CAD build for the part. Positions are in the model's coordinates, mm. A direction names the side the tool comes from. Round coordinates to 2 decimals unless told otherwise and drop trailing zeros. Order: outer loops, then holes, each group sorted by start corner. A loop starts at its lowest first (then second) coordinate and runs counter-clockwise, first axis right, second up. Notation, with made-up numbers: M 11,20 L 15,20 A17 ccw 15,33 Z; hole C -19,72 d7. An arc over 180 degrees is marked long. Answer as a JSON object with one key per item and string values.
```python
from build123d import *

# Parameters (mm, degrees)
EXTRUDE_1_DEPTH     = 100
FILLET_1_R          = 2
SKETCH_2_R          = 2.2
CUT_EXTRUDE_1_DEPTH = 12
CHAMFER_1_SIZE      = 0.4


with BuildPart() as part:
    # Эскиз1 → Бобышка-Вытянуть1 (new body)
    with BuildSketch(Plane.XY):
        Polygon((0, 125), (-36.084391824, 62.5), (-108.253175473, 62.5), (-72.168783649, 0), (-108.253175473, -62.5), (-36.084391824, -62.5), (0, -125), (36.084391824, -62.5), (108.253175473, -62.5), (72.168783649, 0), (108.253175473, 62.5), (36.084391824, 62.5), align=None)
        Polygon((0, 105), (-24.537386441, 62.5), (24.537386441, 62.5), align=None, mode=Mode.SUBTRACT)
        Polygon((-90.932667397, -52.5), (-41.857894516, -52.5), (-66.395280957, -10), align=None, mode=Mode.SUBTRACT)
        Polygon((90.932667397, -52.5), (66.395280957, -10), (41.857894516, -52.5), align=None, mode=Mode.SUBTRACT)
        Polygon((-90.932667397, 52.5), (-41.857894516, 52.5), (-66.395280957, 10), align=None, mode=Mode.SUBTRACT)
        Polygon((90.932667397, 52.5), (66.395280957, 10), (41.857894516, 52.5), align=None, mode=Mode.SUBTRACT)
        Polygon((0, -105), (-24.537386441, -62.5), (24.537386441, -62.5), align=None, mode=Mode.SUBTRACT)
        Polygon((-30.310889132, 52.5), (30.310889132, 52.5), (60.621778265, 0), (30.310889132, -52.5), (-30.310889132, -52.5), (-60.621778265, 0), align=None, mode=Mode.SUBTRACT)
    extrude(amount=EXTRUDE_1_DEPTH)

    # Скругление1
    fillet_1_edges = [part.edges().sort_by_distance(p)[0] for p in [
        (108.253175473, 62.5, 50),
        (108.253175473, -62.5, 50),
        (0, -125, 50),
        (-108.253175473, -62.5, 50),
        (-108.253175473, 62.5, 50),
        (0, 125, 50),
    ]]
    fillet(fillet_1_edges, radius=FILLET_1_R)

    # Эскиз2 → Вырез-Вытянуть1 (cut)
    with BuildSketch(Plane.XY.offset(100)):
        with Locations((0, 115)):
            Circle(SKETCH_2_R)
        with Locations((-99.592921435, -57.5)):
            Circle(SKETCH_2_R)
        with Locations((99.592921435, -57.5)):
            Circle(SKETCH_2_R)
        with Locations((-33.197640478, 57.5)):
            Circle(SKETCH_2_R)
        with Locations((33.197640478, 57.5)):
            Circle(SKETCH_2_R)
        with Locations(Location((-99.592921435, 57.5, 0), (0, 0, 180))):
            Circle(SKETCH_2_R)
        with Locations(Location((99.592921435, 57.5, 0), (0, 0, 180))):
            Circle(SKETCH_2_R)
        with Locations(Location((33.197640478, -57.5, 0), (0, 0, 180))):
            Circle(SKETCH_2_R)
        with Locations(Location((-33.197640478, -57.5, 0), (0, 0, 180))):
            Circle(SKETCH_2_R)
        with Locations(Location((0, -115, 0), (0, 0, 180))):
            Circle(SKETCH_2_R)
        with Locations((-66.395280957, 0)):
            Circle(SKETCH_2_R)
        with Locations((66.395280957, 0)):
            Circle(SKETCH_2_R)
    extrude(amount=-CUT_EXTRUDE_1_DEPTH, mode=Mode.SUBTRACT)

    # Фаска1
    chamfer_1_edges = [part.edges().sort_by_distance(p)[0] for p in [
        (-2.2, 115, 100),
        (64.195280957, 0, 100),
        (-68.595280957, 0, 100),
        (2.2, -115, 100),
        (-101.792921435, -57.5, 100),
        (97.392921435, -57.5, 100),
        (-35.397640478, 57.5, 100),
        (30.997640478, 57.5, 100),
        (-97.392921435, 57.5, 100),
        (101.792921435, 57.5, 100),
        (35.397640478, -57.5, 100),
        (-30.997640478, -57.5, 100),
    ]]
    chamfer(chamfer_1_edges, length=CHAMFER_1_SIZE)


solid = part.part
```
Item 1: Drop flat-ended pins along their axis: pin 1 Ø8 at (x, z) = (-21.5, 44) entering from -Y; pin 2 Ø1.5 at (x, z) = (27.5, 71) entering from +Y; pin 3 Ø14.5 at (x, z) = (11, 44) entering from +Y. Give the stop position or say it passes through.
Worked answers:
{"pin 1": "stops at y = -94.69", "pin 2": "stops at y = 78.67", "pin 3": "stops at y = 118.5"}
Item 2: Saw through at B-B on x = -52. List the corners of the cut face in (y, z).
Worked answers:
{"outline": "M -62.5,0 L -52.5,0 L -52.5,100 L -62.5,100 Z; M -34.93,0 L -14.93,0 L -14.93,100 L -34.93,100 Z; M 14.93,0 L 34.93,0 L 34.93,100 L 14.93,100 Z; M 52.5,0 L 62.5,0 L 62.5,100 L 52.5,100 Z"}
Item 3: Saw through at D-D on z = 65. State how many separate pieces and enclosed holes the cut face has, and give its area (3 significant figures).
Worked answers:
{"separate pieces": "1", "enclosed holes": "7", "area": "11,200 mm2"}
Item 4: Two-plate mould, pull along X, no slides. Class faces 1 (the flat face through (-12.097, -84.048, 49.3)), 2 (the flat face through (-53.955, -31.548, 49.3)), 3 (the flat face through (-40, 37, 100)), 4 (the flat face through (-19.15, -91.83, 49.3)): released by +X, released by -X, zero draft, split by the parting line, or undercut.
Worked answers:
{"face 1": "undercut", "face 2": "undercut", "face 3": "zero draft", "face 4": "released by -X"}
Item 5: Saw through at C-C on y = -13. List the corners of the cut face in (x, z), and give its area (3 significant figures).
Worked answers:
{"outline": "M -79.67,0 L -68.13,0 L -68.13,100 L -79.67,100 Z; M -64.66,0 L -53.12,0 L -53.12,100 L -64.66,100 Z; M 53.12,0 L 64.66,0 L 64.66,100 L 53.12,100 Z; M 68.13,0 L 79.67,0 L 79.67,100 L 68.13,100 Z", "area": "4,620 mm2"}
Item 6: Saw through at A-A on y = 87.5. List the corners of the cut face in (x, z), and give its area (3 significant figures).
Worked answers:
{"outline": "M -21.65,0 L -10.1,0 L -10.1,100 L -21.65,100 Z; M 10.1,0 L 21.65,0 L 21.65,100 L 10.1,100 Z", "area": "2,310 mm2"}
Item 7: Wall check: line 1 along Y through (x, z) = (-46, 21.5); line 2 along Y through (x, z) = (-87.5, 15); line 3 along X through (y, z) = (-47, 44.5). Give the ranges that are in metal, low to high. Write a range as [from, to].
Worked answers:
{"line 1": "y = [-62.5, -52.5], [-45.33, -25.33], [25.33, 45.33], [52.5, 62.5]", "line 2": "y = [-62.5, -52.5], [-46.55, -26.55], [26.55, 46.55], [52.5, 62.5]", "line 3": "x = [-99.3, -87.76], [-45.03, -33.49], [33.49, 45.03], [87.76, 99.3]"}
Item 8: 3-axis set-ups, long thin cutter, end or side, ignore diameter. For faces 5 (the flat face through (18.668, -92.666, 49.3)), 6 (the flat face through (66, -52.5, 49)), 7 (the flat face through (-89.585, 30.167, 49.3)): which of +Z, -Z, +X, -X, +Y, -Y reach the whole face in a straight line?
Worked answers:
{"face 5": "+Z, -Z, +X, -Y", "face 6": "+Z, -Z", "face 7": "+Z, -Z, -X"}
